from build123d import *

# Parameters (mm, degrees)
F0_R     = 1.7399
F0_R_2   = 4
F1_DEPTH = 6.35


with BuildPart() as f1:
    # F0 (on Right) → F1 (new body)
    with BuildSketch(Plane.YZ):
        with BuildLine():
            ThreePointArc((-203.2, -23.014367), (-201.340128, -27.504495), (-196.85, -29.364367))
            Line((-196.85, -29.364367), (-76.2, -29.364367))
            Line((-76.2, -29.364367), (196.85, -29.364367))
            ThreePointArc((196.85, -29.364367), (201.340128, -27.504495), (203.2, -23.014367))
            Line((203.2, -23.014367), (203.2, 23.014367))
            ThreePointArc((203.2, 23.014367), (201.340128, 27.504495), (196.85, 29.364367))
            Line((196.85, 29.364367), (-76.2, 29.364367))
            Line((-76.2, 29.364367), (-196.85, 29.364367))
            ThreePointArc((-196.85, 29.364367), (-201.340128, 27.504495), (-203.2, 23.014367))
            Line((-203.2, 23.014367), (-203.2, -23.014367))
        make_face()
        with Locations((-196.85, -23.014367)):
            Circle(F0_R, mode=Mode.SUBTRACT)
        with BuildLine():
            ThreePointArc((-74.4601, -23.014367), (-74.969705, -24.244662), (-76.2, -24.754267))
            ThreePointArc((-76.2, -24.754267), (-77.430295, -21.784071), (-74.4601, -23.014367))
        make_face(mode=Mode.SUBTRACT)
        with Locations((-139.7, 0)):
            Circle(F0_R_2, mode=Mode.SUBTRACT)
        with BuildLine():
            Line((-34.925, -15.875), (-104.775, -15.875))
            ThreePointArc((-104.775, -15.875), (-119.38, -1.27), (-104.775, 13.335))
            Line((-104.775, 13.335), (-34.925, 13.335))
            ThreePointArc((-34.925, 13.335), (-20.32, -1.27), (-34.925, -15.875))
        make_face(mode=Mode.SUBTRACT)
        Circle(F0_R_2, mode=Mode.SUBTRACT)
        with Locations((76.2, -23.014367)):
            Circle(F0_R, mode=Mode.SUBTRACT)
        with Locations((196.85, -23.014367)):
            Circle(F0_R, mode=Mode.SUBTRACT)
        with BuildLine():
            Line((104.775, -15.875), (34.925, -15.875))
            ThreePointArc((34.925, -15.875), (20.32, -1.27), (34.925, 13.335))
            Line((34.925, 13.335), (104.775, 13.335))
            ThreePointArc((104.775, 13.335), (119.38, -1.27), (104.775, -15.875))
        make_face(mode=Mode.SUBTRACT)
        with Locations((139.7, 0)):
            Circle(F0_R_2, mode=Mode.SUBTRACT)
        with Locations((-196.85, 23.014367)):
            Circle(F0_R, mode=Mode.SUBTRACT)
        with BuildLine():
            ThreePointArc((-74.4601, 23.014367), (-77.430295, 21.784071), (-76.2, 24.754267))
            ThreePointArc((-76.2, 24.754267), (-74.969705, 24.244662), (-74.4601, 23.014367))
        make_face(mode=Mode.SUBTRACT)
        with Locations((76.2, 23.014367)):
            Circle(F0_R, mode=Mode.SUBTRACT)
        with Locations((196.85, 23.014367)):
            Circle(F0_R, mode=Mode.SUBTRACT)
    extrude(amount=F1_DEPTH)


solid = f1.part
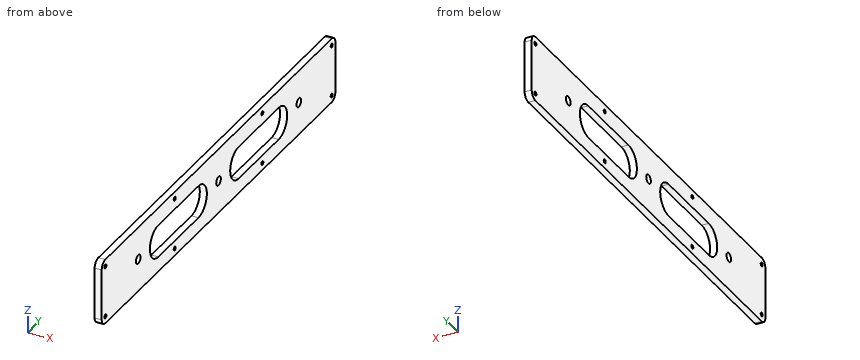
Input: part model. Units: mm. Frame: model coordinates. Round coordinates to 2 decimals unless told otherwise and drop trailing zeros. Write each loop counter-clockwise with the first axis right and the second up, starting at its lowest first coordinate (ties: lowest second). Pieces come first, ordered by that corner, then holes.
1) Cut plane D-D (y = -139.7). Return the cut outline in (x, z).
2) Cut plane A-A (y = 42.5). Return the cut outline in (x, z) (3 decimals).
3) Cut plane C-C (z = 0). Return the cut outline in (x, y).
4) Contact query for flat-ended pins moving along their axis: P1, Ø10.5, axis at y = 0, z = 0, coming from the -X side; P2, Ø2, axis at y = 196.85, z = -23.01, coming from the +X side. Output: stop coordinate, or through.
5) Cut plane B-B (x = 2). Count the separate pieces of the cut face and the enclosed holes in it, then the cut area to 3 significant figures.
6) Ray query, L1, parallel to Z at x = 2, y = -76.2 (3 decimals); L2, parallel to Y at x = 3.75, z = -23; L3, parallel to Z at x = 1.5, y = 196.85. Return the intervals inside material, ascending.
Geometry says:
1. outline: (0, -29.36) - (6.35, -29.36) - (6.35, -4) - (0, -4) - close; (0, 4) - (6.35, 4) - (6.35, 29.36) - (0, 29.36) - close
2. outline: (0, -29.364) - (6.35, -29.364) - (6.35, -15.875) - (0, -15.875) - close; (0, 13.335) - (6.35, 13.335) - (6.35, 29.364) - (0, 29.364) - close
3. outline: (0, -203.2) - (6.35, -203.2) - (6.35, -143.7) - (0, -143.7) - close; (0, -135.7) - (6.35, -135.7) - (6.35, -119.32) - (0, -119.32) - close; (0, -20.38) - (6.35, -20.38) - (6.35, -4) - (0, -4) - close; (0, 4) - (6.35, 4) - (6.35, 20.38) - (0, 20.38) - close; (0, 119.32) - (6.35, 119.32) - (6.35, 135.7) - (0, 135.7) - close; (0, 143.7) - (6.35, 143.7) - (6.35, 203.2) - (0, 203.2) - close
4. P1: stops at x = 0
4. P2: passes through
5. separate pieces: 1
5. enclosed holes: 13
5. area: 18,200 mm2
6. L1: z = -29.364 to -24.754, -21.274 to -15.875, 13.335 to 21.274, 24.754 to 29.364
6. L2: y = -203.2 to -198.59, -195.11 to -77.94, -74.46 to 74.46, 77.94 to 195.11, 198.59 to 203.2
6. L3: z = -29.36 to -24.75, -21.27 to 21.27, 24.75 to 29.36
